from build123d import *
from build123d.topology import SkipClean

# Parameters (mm, degrees)
EXTRUDE_1_DEPTH     = 3.5
EXTRUDE_START       = 3
SKETCH_2_R          = 1.7
EXTRUDE_2_DEPTH     = 3
SKETCH_3_R          = 0.75
CUT_EXTRUDE_1_DEPTH = 88.945086175
SKETCH_4_R          = 12
CUT_EXTRUDE_2_DEPTH = 88.945086175
CUT_EXTRUDE_START   = -1
SKETCH_5_R          = 1.75
SKETCH_5_R_2        = 0.75
CUT_EXTRUDE_4_DEPTH = 1
SKETCH_6_W          = 3
SKETCH_6_H          = 50
CUT_EXTRUDE_5_DEPTH = 100.398968375


with BuildPart() as part:
    # 草图1 → 凸台-拉伸1 (new body)
    with BuildSketch(Plane.XY):
        with BuildLine():
            ThreePointArc((31.968716166, 26.753538627), (7.644242894, 16.6780119), (-2.431283834, -7.646461373))
            ThreePointArc((-2.431283834, -7.646461373), (31.968716166, -42.046461373), (66.368716166, -7.646461373))
            ThreePointArc((66.368716166, -7.646461373), (56.293189439, 16.6780119), (31.968716166, 26.753538627))
        make_face()
        with BuildLine():
            ThreePointArc((7.286992159, 4.903538627), (8.986992159, 6.603538627), (7.286992159, 8.303538627))
            ThreePointArc((7.286992159, 8.303538627), (5.586992159, 6.603538627), (7.286992159, 4.903538627))
        make_face(mode=Mode.SUBTRACT)
        with BuildLine():
            ThreePointArc((56.650440174, 8.303538627), (54.950440174, 6.603538627), (56.650440174, 4.903538627))
            ThreePointArc((56.650440174, 4.903538627), (58.350440174, 6.603538627), (56.650440174, 8.303538627))
        make_face(mode=Mode.SUBTRACT)
        with BuildLine():
            ThreePointArc((7.286992159, -23.596461373), (8.986992159, -21.896461373), (7.286992159, -20.196461373))
            ThreePointArc((7.286992159, -20.196461373), (5.586992159, -21.896461373), (7.286992159, -23.596461373))
        make_face(mode=Mode.SUBTRACT)
        with BuildLine():
            ThreePointArc((56.650440174, -20.196461373), (54.950440174, -21.896461373), (56.650440174, -23.596461373))
            ThreePointArc((56.650440174, -23.596461373), (58.350440174, -21.896461373), (56.650440174, -20.196461373))
        make_face(mode=Mode.SUBTRACT)
    extrude(amount=EXTRUDE_1_DEPTH)

    # 草图2 → 凸台-拉伸2 (add)
    # profile 1 of 3: a face of its own
    with SkipClean():  # the faces are left unmerged after this step: merging them gives an invalid solid
        with BuildSketch(Plane(origin=(0, 0, 0), x_dir=(-1, 0, 0), z_dir=(0, 0, -1)).offset(EXTRUDE_START)):
            with BuildLine():
                ThreePointArc((-55.598358567, 17.353538627), (-66.368716166, -7.646461373), (-55.598358567, -32.646461373))
                Line((-55.598358567, -32.646461373), (-8.339073765, -32.646461373))
                ThreePointArc((-8.339073765, -32.646461373), (-0.375839607, -21.257124498), (2.431283834, -7.646461373))
                ThreePointArc((2.431283834, -7.646461373), (-0.375839607, 5.964201752), (-8.339073765, 17.353538627))
                Line((-8.339073765, 17.353538627), (-55.598358567, 17.353538627))
            make_face()
            with Locations((-56.650440174, -21.896461373)):
                Circle(SKETCH_2_R, mode=Mode.SUBTRACT)
            with Locations((-7.286992159, -21.896461373)):
                Circle(SKETCH_2_R, mode=Mode.SUBTRACT)
            with Locations((-56.650440174, 6.603538627)):
                Circle(SKETCH_2_R, mode=Mode.SUBTRACT)
            with Locations((-7.286992159, 6.603538627)):
                Circle(SKETCH_2_R, mode=Mode.SUBTRACT)
        # profile 2 of 3: a face of its own
        with BuildSketch(Plane(origin=(0, 0, 0), x_dir=(-1, 0, 0), z_dir=(0, 0, -1)).offset(EXTRUDE_START)):
            with BuildLine():
                Line((-76.968716166, 17.353538627), (-76.968716166, -32.646461373))
                Line((-76.968716166, -32.646461373), (-55.598358567, -32.646461373))
                ThreePointArc((-55.598358567, -32.646461373), (-66.368716166, -7.646461373), (-55.598358567, 17.353538627))
                Line((-55.598358567, 17.353538627), (-76.968716166, 17.353538627))
            make_face()
        # profile 3 of 3: a face of its own
        with BuildSketch(Plane(origin=(0, 0, 0), x_dir=(-1, 0, 0), z_dir=(0, 0, -1)).offset(EXTRUDE_START)):
            with BuildLine():
                ThreePointArc((2.431283834, -7.646461373), (-0.375839607, -21.257124498), (-8.339073765, -32.646461373))
                Line((-8.339073765, -32.646461373), (13.031283834, -32.646461373))
                Line((13.031283834, -32.646461373), (13.031283834, 17.353538627))
                Line((13.031283834, 17.353538627), (-8.339073765, 17.353538627))
                ThreePointArc((-8.339073765, 17.353538627), (-0.375839607, 5.964201752), (2.431283834, -7.646461373))
            make_face()
        extrude(amount=-EXTRUDE_2_DEPTH)

    # 草图3 → 切除-拉伸1 (cut, through all)
    with SkipClean():  # the faces are left unmerged after this step: merging them gives an invalid solid
        with BuildSketch(Plane(origin=(0, 0, -3), x_dir=(-1, 0, 0), z_dir=(0, 0, -1))):
            with Locations((-47.468716166, 7.853538627)):
                Circle(SKETCH_3_R)
            with Locations(Location((-47.468716166, -23.146461373, 0), (0, 0, 180))):
                Circle(SKETCH_3_R)
            with Locations(Location((-16.468716166, 7.853538627, 0), (0, 0, 180))):
                Circle(SKETCH_3_R)
            with Locations((-16.468716166, -23.146461373)):
                Circle(SKETCH_3_R)
            with Locations((-53.968716166, 14.353538627)):
                Circle(SKETCH_3_R)
            with Locations(Location((-53.968716166, -29.646461373, 0), (0, 0, 180))):
                Circle(SKETCH_3_R)
            with Locations((-9.968716166, -29.646461373)):
                Circle(SKETCH_3_R)
            with Locations(Location((-9.968716166, 14.353538627, 0), (0, 0, 180))):
                Circle(SKETCH_3_R)
        extrude(amount=-CUT_EXTRUDE_1_DEPTH, mode=Mode.SUBTRACT)

    # 草图4 → 切除-拉伸2 (cut, through all)
    with SkipClean():  # the faces are left unmerged after this step: merging them gives an invalid solid
        with BuildSketch(Plane.XY.offset(3.5)):
            with Locations((31.968716166, -7.646461373)):
                Circle(SKETCH_4_R)
        extrude(amount=-CUT_EXTRUDE_2_DEPTH, mode=Mode.SUBTRACT)

    # 草图5 → 切除-拉伸4 (cut)
    # profile 1 of 8: a face of its own
    with SkipClean():  # the faces are left unmerged after this step: merging them gives an invalid solid
        with BuildSketch(Plane.XY.offset(3.5).offset(CUT_EXTRUDE_START)):
            with Locations((9.968716166, 14.353538627)):
                Circle(SKETCH_5_R)
            with Locations((9.968716166, 14.353538627)):
                Circle(SKETCH_5_R_2, mode=Mode.SUBTRACT)
        # profile 2 of 8: a face of its own
        with BuildSketch(Plane.XY.offset(3.5).offset(CUT_EXTRUDE_START)):
            with Locations((16.468716166, 7.853538627)):
                Circle(SKETCH_5_R)
            with Locations((16.468716166, 7.853538627)):
                Circle(SKETCH_5_R_2, mode=Mode.SUBTRACT)
        # profile 3 of 8: a face of its own
        with BuildSketch(Plane.XY.offset(3.5).offset(CUT_EXTRUDE_START)):
            with Locations((47.468716166, 7.853538627)):
                Circle(SKETCH_5_R)
            with Locations(Location((47.468716166, 7.853538627, 0), (0, 0, 180))):
                Circle(SKETCH_5_R_2, mode=Mode.SUBTRACT)
        # profile 4 of 8: a face of its own
        with BuildSketch(Plane.XY.offset(3.5).offset(CUT_EXTRUDE_START)):
            with Locations((53.968716166, 14.353538627)):
                Circle(SKETCH_5_R)
            with Locations(Location((53.968716166, 14.353538627, 0), (0, 0, 180))):
                Circle(SKETCH_5_R_2, mode=Mode.SUBTRACT)
        # profile 5 of 8: a face of its own
        with BuildSketch(Plane.XY.offset(3.5).offset(CUT_EXTRUDE_START)):
            with Locations((47.468716166, -23.146461373)):
                Circle(SKETCH_5_R)
            with Locations((47.468716166, -23.146461373)):
                Circle(SKETCH_5_R_2, mode=Mode.SUBTRACT)
        # profile 6 of 8: a face of its own
        with BuildSketch(Plane.XY.offset(3.5).offset(CUT_EXTRUDE_START)):
            with Locations((16.468716166, -23.146461373)):
                Circle(SKETCH_5_R)
            with Locations(Location((16.468716166, -23.146461373, 0), (0, 0, 180))):
                Circle(SKETCH_5_R_2, mode=Mode.SUBTRACT)
        # profile 7 of 8: a face of its own
        with BuildSketch(Plane.XY.offset(3.5).offset(CUT_EXTRUDE_START)):
            with Locations((9.968716166, -29.646461373)):
                Circle(SKETCH_5_R)
            with Locations(Location((9.968716166, -29.646461373, 0), (0, 0, 180))):
                Circle(SKETCH_5_R_2, mode=Mode.SUBTRACT)
        # profile 8 of 8: a face of its own
        with BuildSketch(Plane.XY.offset(3.5).offset(CUT_EXTRUDE_START)):
            with Locations((53.968716166, -29.646461373)):
                Circle(SKETCH_5_R)
            with Locations((53.968716166, -29.646461373)):
                Circle(SKETCH_5_R_2, mode=Mode.SUBTRACT)
        extrude(amount=CUT_EXTRUDE_4_DEPTH, mode=Mode.SUBTRACT)

    # 草图6 → 切除-拉伸5 (cut, through all)
    with BuildSketch(Plane(origin=(76.968716166, 0, 0), x_dir=(0, 0, -1), z_dir=(1, 0, 0))):
        with Locations((1.5, -7.646461373)):
            Rectangle(SKETCH_6_W, SKETCH_6_H)
    extrude(amount=-CUT_EXTRUDE_5_DEPTH, mode=Mode.SUBTRACT)


solid = part.part
Verification items for the finished model (mm, model axes). A direction names the side the tool comes from. Round coordinates to 2 decimals unless told otherwise and drop trailing zeros. Loops run counter-clockwise (first coordinate to the right, second up) from the corner with the lowest first, then second, coordinate; pieces in that order, holes last. Notation, with made-up numbers: (-33, -28.75) - (-29, -28.75) arc R27 ccw to (-29, 3.25) - close; hole circle Ø2 at (40, -21). An arc over 180 degrees is marked (long way). Answer in a Markdown table with one row per item. Add a question column.
Q1. Section check B-B on y = -12.5. Enter the section's corners in (x, z), plus the area to 3 significant figures.
Q2. Section check A-A on x = 42.5. Enter the section's corners in (y, z).
Q3. Gauge pin test, flat ends, axial feed: pin 1 (1.7 mm diameter, centred on x = 9.5, y = 14, fed in from +Z); pin 2 (19 mm diameter, centred on x = 31.97, y = -7.65, fed in from -Z); pin 3 (1 mm diameter, centred on x = 41.5, z = 3, fed in from +Y); pin 4 (1.5 mm diameter, centred on x = 9, z = 2.5, fed in from +Y). Record the tip position at first contact, or that the pin passes through.
Q4. Section check D-D on x = 62. Enter the section's corners in (y, z).
Q5. Section check C-C on z = 0.9. State how many separate pieces and enclosed holes the cut face has, plus the area to 3 significant figures.
Q6. Tool access check on faces 1 (the face through (53.276, 14.066, 1.232)), 2 (the face through (53.589, -31.355, 2.993)). Record the directions out of +Z, -Z, +X, -X, +Y, -Y that give a thin tool (end or side, any length) a straight path to the whole face; none if there is none.
Q7. Material ranges on line 1 (X direction, y = -29.5, z = 0.6); line 2 (X direction, y = 8.5, z = 1.6); line 3 (Y direction, x = 8.5, z = 0.6), recorded low to high.
Found:
| question | item | result |
|---|---|---|
| 1 | outline | (-2.09, 0) - (20.99, 0) - (20.99, 3.5) - (-2.09, 3.5) - close; (42.94, 0) - (66.02, 0) - (66.02, 3.5) - (42.94, 3.5) - close |
| 1 | area | 162 mm² |
| 2 | outline | (-40.39, 0) - (-13.4, 0) - (-13.4, 3.5) - (-40.39, 3.5) - close; (-1.89, 0) - (25.1, 0) - (25.1, 3.5) - (-1.89, 3.5) - close |
| 3 | pin 1 | stops at z = 2.5 |
| 3 | pin 2 | passes through |
| 3 | pin 3 | stops at y = 25.55 |
| 3 | pin 4 | stops at y = 18.62 |
| 4 | outline | (-24.42, 0) - (9.13, 0) - (9.13, 3.5) - (-24.42, 3.5) - close |
| 5 | separate pieces | 1 |
| 5 | enclosed holes | 13 |
| 5 | area | 3,210 mm² |
| 6 | face 1 | +Z, -Z |
| 6 | face 2 | +Z |
| 7 | line 1 | x = 5.4 to 9.23, 10.7 to 53.23, 54.7 to 58.54 |
| 7 | line 2 | x = 1.59 to 16.09, 16.85 to 47.09, 47.85 to 62.34 |
| 7 | line 3 | y = -32.8 to -23.09, -20.71 to 5.41, 7.79 to 17.5 |
